from build123d import *

# Parameters (mm, degrees)
BOSS_EXTRUDE1_DEPTH     = 20
SKETCH3_R               = 36
BOSS_EXTRUDE2_DEPTH     = 30
BOSS_EXTRUDE3_DEPTH     = 8
SKETCH6_W               = 30
SKETCH6_H               = 8
SKETCH6_W_2             = 20
CUT_EXTRUDE1_DEPTH      = 92
CUT_EXTRUDE1_DEPTH_BACK = 92
SKETCH7_R               = 15
CUT_EXTRUDE2_DEPTH      = 51
CUT_EXTRUDE2_DEPTH_BACK = 1


with BuildPart() as part:
    # Sketch2 → Boss-Extrude1 (new body)
    with BuildSketch(Plane(origin=(0, 0, 0), x_dir=(1, 0, 0), z_dir=(0, 1, 0))):
        with BuildLine():
            Line((-55, 36), (55, 36))
            ThreePointArc((55, 36), (91, 0), (55, -36))
            Line((55, -36), (-55, -36))
            ThreePointArc((-55, -36), (-91, 0), (-55, 36))
        make_face()
    extrude(amount=BOSS_EXTRUDE1_DEPTH)

    # Sketch3 → Boss-Extrude2 (add)
    with BuildSketch(Plane(origin=(0, 20, 0), x_dir=(1, 0, 0), z_dir=(0, 1, 0))):
        with Locations((-55, 0)):
            Circle(SKETCH3_R)
    extrude(amount=BOSS_EXTRUDE2_DEPTH)

    # Sketch4 → Boss-Extrude3 (add)
    with BuildSketch(Plane(origin=(0, 20, 0), x_dir=(1, 0, 0), z_dir=(0, 1, 0))):
        with BuildLine():
            Line((18.5, 20), (53.5, 20))
            ThreePointArc((53.5, 20), (73.5, 0), (53.5, -20))
            Line((53.5, -20), (18.5, -20))
            ThreePointArc((18.5, -20), (-1.5, 0), (18.5, 20))
        make_face()
    extrude(amount=BOSS_EXTRUDE3_DEPTH)

    # Sketch6 → Cut-Extrude1 (cut, two sides)
    with BuildSketch(Plane(origin=(0, 0, 0), x_dir=(0, 0, -1), z_dir=(1, 0, 0))) as cut_extrude1_sk:
        with Locations((0, 4)):
            Rectangle(SKETCH6_W, SKETCH6_H)
        with Locations((0, 46)):
            Rectangle(SKETCH6_W_2, SKETCH6_H)
    extrude(amount=CUT_EXTRUDE1_DEPTH, mode=Mode.SUBTRACT)
    extrude(cut_extrude1_sk.sketch, amount=-CUT_EXTRUDE1_DEPTH_BACK, mode=Mode.SUBTRACT)

    # Sketch7 → Cut-Extrude2 (cut, two sides)
    with BuildSketch(Plane(origin=(0, 0, 0), x_dir=(1, 0, 0), z_dir=(0, 1, 0))) as cut_extrude2_sk:
        with Locations((-55, 0)):
            Circle(SKETCH7_R)
        with BuildLine():
            Line((18.5, 10), (53.5, 10))
            ThreePointArc((53.5, 10), (63.5, 0), (53.5, -10))
            Line((53.5, -10), (18.5, -10))
            ThreePointArc((18.5, -10), (8.5, 0), (18.5, 10))
        make_face()
    extrude(amount=CUT_EXTRUDE2_DEPTH, mode=Mode.SUBTRACT)
    extrude(cut_extrude2_sk.sketch, amount=-CUT_EXTRUDE2_DEPTH_BACK, mode=Mode.SUBTRACT)


solid = part.part
Can you work these out from the model? Positions are in its coordinate system, mm. A direction names the side the tool comes from. Give positions to 0.01 mm unless a question says otherwise; leave off trailing zeros. Loops run counter-clockwise (first coordinate to the right, second up) from the corner with the lowest first, then second, coordinate; pieces in that order, holes last. Notation, with made-up numbers: (14.25, 10) - (19.25, 10) arc R21 ccw to (19.25, 37) - close; hole circle Ø10 at (-34, 32.5). An arc over 180 degrees is marked (long way). One line per item, written item: value.
(1) If we section it at B-B, the plane y = 24.5: List the corners of the cut face in (x, z) for me, plus the area to 3 significant figures.
Verdict:
outline: circle Ø72 at (-55, 0); (18.5, -20) - (53.5, -20) arc R20 ccw to (53.5, 20) - (18.5, 20) arc R20 ccw to start; hole circle Ø30 at (-55, 0); hole (18.5, -10) - (53.5, -10) arc R10 ccw to (53.5, 10) - (18.5, 10) arc R10 ccw to start
area: 5,010 mm^2
(2) If we section it at D-D, the plane y = 45.5: List the corners of the cut face in (x, z) for me, plus the area to 3 significant figures.
Verdict:
outline: (-89.58, -10) arc R36 ccw to (-20.42, -10) - (-43.82, -10) arc R15 cw to (-66.18, -10) - close; (-89.58, 10) - (-66.18, 10) arc R15 cw to (-43.82, 10) - (-20.42, 10) arc R36 ccw to start
area: 2,500 mm^2
(3) If we section it at A-A, the plane z = 0: List the corners of the cut face in (x, y) for me.
Verdict:
outline: (-91, 8) - (-70, 8) - (-70, 42) - (-91, 42) - close; (-40, 8) - (8.5, 8) - (8.5, 28) - (-1.5, 28) - (-1.5, 20) - (-19, 20) - (-19, 42) - (-40, 42) - close; (63.5, 8) - (91, 8) - (91, 20) - (73.5, 20) - (73.5, 28) - (63.5, 28) - close
(4) If we section it at C-C, the plane x = 43.5: List the corners of the cut face in (y, z) for me.
Verdict:
outline: (0, -36) - (20, -36) - (20, -20) - (28, -20) - (28, -10) - (8, -10) - (8, -15) - (0, -15) - close; (0, 15) - (8, 15) - (8, 10) - (28, 10) - (28, 20) - (20, 20) - (20, 36) - (0, 36) - close
(5) I'm going to push flat-ended pins straight in: pin 1 (24 mm diameter, centred on x = -20, z = 1.5, fed in from -Y); pin 2 (2.5 mm diameter, centred on x = -37, y = 46, fed in from +Z); pin 3 (2.5 mm diameter, centred on x = -74, y = 3.5, fed in from +Z). Where does each tip first touch, or does it pass through?
Verdict:
pin 1: y = 8
pin 2: z = 31.87
pin 3: z = 31.32
(6) I need wall thicknesses on line 1 along X through (y, z) = (27, 0); line 2 along X through (y, z) = (17, 0); line 3 along X through (y, z) = (33.5, -0.5). Which ranges of each line are inside material? Lowest first, please.
Verdict:
line 1: -91 to -70, -40 to -19, -1.5 to 8.5, 63.5 to 73.5
line 2: -91 to -70, -40 to 8.5, 63.5 to 91
line 3: -91 to -69.99, -40.01 to -19
(7) If we mould it in two halves opening along X, with no side actions, what happens to faces 1 (the face through (8.5, 17.9, 0.2)), 2 (the face through (-55, 50, 20)), 3 (the face through (90.99, 9.86, -0.79))? For each: released by +X, released by -X, zero draft, split by the parting line, or undercut.
Verdict:
face 1: undercut
face 2: zero draft
face 3: released by +X
(8) On a 3-axis mill with a long thin cutter (end or side, diameter ignored), from which of +Z, -Z, +X, -X, +Y, -Y can I reach the whole of each face in a straight line? I mean faces 4 (the face through (-77, 8, 0)), 5 (the face through (37, 28, -14)), 6 (the face through (36, 24, -20)), 7 (the face through (-32, 46, 10)), 8 (the face through (36, 18, -10)). Say none if no direction works.
Verdict:
face 4: +X, -X, -Y
face 5: +Z, -Z, +X, +Y
face 6: -Z, +X, +Y
face 7: +X, -X, +Y
face 8: +Y, -Y
